```python
from build123d import *

# Parameters (mm, degrees)
F0_R     = 4.5
F1_DEPTH = 3


# Not quite as in the source:
# - ends of sketch curves that miss each other by under 0.0002 mm in the source are joined


with BuildPart() as f1:
    # F0 (on Front) → F1 (new body)
    with BuildSketch(Plane.XZ):
        with BuildLine():
            ThreePointArc((-123.4212349358, 88.5414632024), (-130.4923027477, 85.6125310143), (-133.4212349358, 78.5414632024))
            Line((-133.4212349358, 78.5414632024), (-133.4212349358, -66.4585367976))
            ThreePointArc((-133.4212349358, -66.4585367976), (-130.4923027477, -73.5296046095), (-123.4212349358, -76.4585367976))
            Line((-123.4212349358, -76.4585367976), (36.5787650642, -76.4585367976))
            ThreePointArc((36.5787650642, -76.4585367976), (43.6498328761, -73.5296046095), (46.5787650642, -66.4585367976))
            Line((46.5787650642, -66.4585367976), (46.5787650642, 78.5414632024))
            ThreePointArc((46.5787650642, 78.5414632024), (43.6498328761, 85.6125310143), (36.5787650642, 88.5414632024))
            Line((36.5787650642, 88.5414632024), (-123.4212349358, 88.5414632024))
        make_face()
        with Locations((-116.9212349358, -66.9585367976)):
            Circle(F0_R, mode=Mode.SUBTRACT)
        with Locations((-116.9212349358, -42.9585367976)):
            Circle(F0_R, mode=Mode.SUBTRACT)
        with BuildLine():
            Line((-80.7012349358, -46.4585367976), (-80.7012349358, -61.4585367976))
            ThreePointArc((-80.7012349358, -61.4585367976), (-82.2012349358, -62.9585367976), (-83.7012349358, -61.4585367976))
            Line((-83.7012349358, -61.4585367976), (-83.7012349358, -46.4585367976))
            ThreePointArc((-83.7012349358, -46.4585367976), (-82.2012349358, -44.9585367976), (-80.7012349358, -46.4585367976))
        make_face(mode=Mode.SUBTRACT)
        with BuildLine():
            ThreePointArc((-3.0212349358, -61.4585367976), (-4.5212349358, -62.9585367976), (-6.0212349358, -61.4585367976))
            Line((-6.0212349358, -61.4585367976), (-6.0212349358, -46.4585367976))
            ThreePointArc((-6.0212349358, -46.4585367976), (-4.5212349358, -44.9585367976), (-3.0212349358, -46.4585367976))
            Line((-3.0212349358, -46.4585367976), (-3.0212349358, -61.4585367976))
        make_face(mode=Mode.SUBTRACT)
        with Locations((34.5787650642, -66.9585362183)):
            Circle(F0_R, mode=Mode.SUBTRACT)
        with Locations((34.5787650642, -42.9585362183)):
            Circle(F0_R, mode=Mode.SUBTRACT)
        with BuildLine():
            ThreePointArc((-8, -34.2985367976), (-9.5, -32.7985367976), (-8, -31.2985367976))
            Line((-8, -31.2985367976), (7, -31.2985367976))
            ThreePointArc((7, -31.2985367976), (8.5, -32.7985367976), (7, -34.2985367976))
            Line((7, -34.2985367976), (0, -34.2985367976))
            Line((0, -34.2985367976), (-8, -34.2985367976))
        make_face(mode=Mode.SUBTRACT)
        with BuildLine():
            ThreePointArc((22, -33.4585367976), (20.5, -31.9585367976), (22, -30.4585367976))
            Line((22, -30.4585367976), (37, -30.4585367976))
            ThreePointArc((37, -30.4585367976), (38.5, -31.9585367976), (37, -33.4585367976))
            Line((37, -33.4585367976), (22, -33.4585367976))
        make_face(mode=Mode.SUBTRACT)
        with BuildLine():
            ThreePointArc((-55.3851271454, 21.5414632024), (-53.8851271454, 23.0414632024), (-52.3851271454, 21.5414632024))
            Line((-52.3851271454, 21.5414632024), (-52.3738959134, -3.4585362183))
            ThreePointArc((-52.3738959134, -3.4585362183), (-53.8738959134, -4.9585367976), (-55.3738959134, -3.4585362183))
            Line((-55.3738959134, -3.4585362183), (-55.3851271454, 21.5414632024))
        make_face(mode=Mode.SUBTRACT)
        with Locations((-116.9212349358, 77.0414632024)):
            Circle(F0_R, mode=Mode.SUBTRACT)
        with BuildLine():
            ThreePointArc((-32.8738959134, -3.4585371545), (-34.3738959134, -4.9585367976), (-35.8738959134, -3.4585371545))
            Line((-35.8738959134, -3.4585371545), (-35.8738959134, 21.5414632024))
            ThreePointArc((-35.8738959134, 21.5414632024), (-34.3738959134, 23.0414632024), (-32.8738959134, 21.5414632024))
            Line((-32.8738959134, 21.5414632024), (-32.8738959134, -3.4585371545))
        make_face(mode=Mode.SUBTRACT)
        with BuildLine():
            Line((7, 43.3814632024), (-8, 43.3814632024))
            ThreePointArc((-8, 43.3814632024), (-9.5, 44.8814632024), (-8, 46.3814632024))
            Line((-8, 46.3814632024), (7, 46.3814632024))
            ThreePointArc((7, 46.3814632024), (8.5, 44.8814632024), (7, 43.3814632024))
        make_face(mode=Mode.SUBTRACT)
        with BuildLine():
            Line((22, 45.5414632024), (37, 45.5414632024))
            ThreePointArc((37, 45.5414632024), (38.5, 44.0414632024), (37, 42.5414632024))
            Line((37, 42.5414632024), (22, 42.5414632024))
            ThreePointArc((22, 42.5414632024), (20.5, 44.0414632024), (22, 45.5414632024))
        make_face(mode=Mode.SUBTRACT)
        with Locations((34.5787650642, 77.0414632024)):
            Circle(F0_R, mode=Mode.SUBTRACT)
    extrude(amount=F1_DEPTH)


solid = f1.part
```
Input: part model. Units: mm. Frame: model coordinates. Round coordinates to 2 decimals unless told otherwise and drop trailing zeros. Loops run counter-clockwise (first coordinate to the right, second up) from the corner with the lowest first, then second, coordinate; pieces in that order, holes last. Notation, with made-up numbers: (-15.75, 61.5) -> (1.25, 61.5) arc R22 cw to (1.25, 72.5) -> close; hole circle Ø8 at (33, -38). An arc over 180 degrees is marked (long way). One line per item, written item: value.
(1) Section A-A (x = 5). Return the cut outline in (y, z), plus the area to 3 significant figures.
Geometry check:
outline: (-3, -76.46) -> (0, -76.46) -> (0, -34.3) -> (-3, -34.3) -> close; (-3, -31.3) -> (0, -31.3) -> (0, 43.38) -> (-3, 43.38) -> close; (-3, 46.38) -> (0, 46.38) -> (0, 88.54) -> (-3, 88.54) -> close
area: 477 mm2
(2) Mould query, pull axis Z, two halves, no side actions, for faces 1 (the face through (-45, -3, 7)), 2 (the face through (43.57, -1.48, -73.61)), 3 (the face through (-121.417, -1.479, -66.761)). Classes: pulls with the +Z half, pulls with the -Z half, needs draft (parallel to the pull), parting line crosses it, or undercut.
Geometry check:
face 1: needs draft
face 2: pulls with the -Z half
face 3: undercut
(3) Section B-B (z = 15). Return the cut outline in (x, y).
Geometry check:
outline: (-133.42, -3) -> (-55.38, -3) -> (-55.38, 0) -> (-133.42, 0) -> close; (-52.38, -3) -> (-35.87, -3) -> (-35.87, 0) -> (-52.38, 0) -> close; (-32.87, -3) -> (46.58, -3) -> (46.58, 0) -> (-32.87, 0) -> close
(4) Section C-C (y = -1). Give the number of separate pieces and of enclosed holes in the cut face, plus the area to 3 significant figures.
Geometry check:
separate pieces: 1
enclosed holes: 14
area: 28,800 mm2
(5) Material intervals for line 1 (X direction, y = -0.6, z = -53); line 2 (X direction, y = -2.1, z = 18.5); line 3 (Z direction, x = -3.5, y = -2.1), sorted ascending. Write a range as [from, to].
Geometry check:
line 1: [-133.42, -83.7], [-80.7, -6.02], [-3.02, 46.58]
line 2: [-133.42, -55.38], [-52.38, -35.87], [-32.87, 46.58]
line 3: [-76.46, -62.56], [-45.36, -34.3], [-31.3, 43.38], [46.38, 88.54]
